```python
from build123d import *

# Parameters (mm, degrees)
MASS_DEPTH         = 6.35
SKETCH4_R          = 3.175
CUT_EXTRUDE1_DEPTH = 73.574972012
SKETCH3_W          = 12.7
SKETCH3_H          = 12.7
CUT_EXTRUDE2_DEPTH = 73.574972012
LPATTERN1_COUNT    = 3
LPATTERN1_PITCH    = 25.4


with BuildPart() as part:
    # Sketch1 → Mass (new body)
    with BuildSketch(Plane.XY):
        with BuildLine():
            Line((-44.45, -23.8125), (44.45, -23.8125))
            Line((44.45, -23.8125), (44.45, 23.8125))
            Line((44.45, 23.8125), (-44.45, 23.8125))
            ThreePointArc((-44.45, 23.8125), (-68.2625, 0), (-44.45, -23.8125))
        make_face()
    extrude(amount=MASS_DEPTH)

    # Sketch4 → Cut-Extrude1 (cut, through all)
    with BuildSketch(Plane(origin=(0, 0, 0), x_dir=(-1, 0, 0), z_dir=(0, 0, -1))):
        with Locations((44.45, 0)):
            Circle(SKETCH4_R)
    extrude(amount=-CUT_EXTRUDE1_DEPTH, mode=Mode.SUBTRACT)

    # Sketch3 → Cut-Extrude2 (cut, through all)
    with BuildSketch(Plane(origin=(0, 0, 0), x_dir=(-1, 0, 0), z_dir=(0, 0, -1))):
        with Locations((-25.4, 23.8125)):
            Rectangle(SKETCH3_W, SKETCH3_H)
        with Locations((-25.4, -23.8125)):
            Rectangle(SKETCH3_W, SKETCH3_H)
    cut_extrude2 = extrude(amount=-CUT_EXTRUDE2_DEPTH, mode=Mode.SUBTRACT)

    # LPattern1: Cut-Extrude2 ×3
    with Locations(*[(-i * LPATTERN1_PITCH, 0, 0) for i in range(1, LPATTERN1_COUNT)]):
        add(cut_extrude2, mode=Mode.SUBTRACT)


solid = part.part
```
Check sheet for the modelled part. Datum: model origin and axes. Units: mm. A direction names the side the tool comes from. Round coordinates to 2 decimals unless told otherwise and drop trailing zeros. Loops run counter-clockwise (first coordinate to the right, second up) from the corner with the lowest first, then second, coordinate; pieces in that order, holes last. Notation, with made-up numbers: (84, 82) - (118, 82) arc R15 ccw to (118, 107) - close; hole circle Ø8 at (12.5, -5.5). An arc over 180 degrees is marked (long way). Answer as a JSON object with one key per item and string values. Group by question number.
Q1. Set-up check for faces 1 (the face through (-38, 23.812, 3)), 2 (the face through (0, 17.462, 3)), 3 (the face through (6.35, -21, 3)): record each of +Z, -Z, +X, -X, +Y, -Y from which the full face is reachable in a straight line by a thin tool's end or side.
Q2. Sectioned sample at C-C, the plane x = -43. Enter the section's corners in (y, z), plus the area to 3 significant figures.
Q3. Scan lines: line 1 along Y through (x, z) = (-44.45, 3.75) (1 decimal); line 2 along X through (y, z) = (-21.5, 2.5); line 3 along Y through (x, z) = (23, 2). Record each from-to range of solid material in increasing order. Write a range as [from, to].
Q4. Gauge pin test, flat ends, axial feed: P1, Ø3, axis at x = 24.5, z = 4.5, coming from the +Y side; P2, Ø1.9, axis at y = -21, z = 4, coming from the -X side; P3, Ø3, axis at y = -22, z = 4, coming from the -X side. Record the tip position at first contact, or that the pin passes through.
Q5. Sectioned sample at D-D, the plane y = -18.5. Enter the section's corners in (x, z).
Q6. Mould release check, pull along X, two halves, no side actions. Record for faces 4 (the face through (-13, 0, 0)), 5 (the face through (-19.05, 21, 3)), 6 (the face through (-68.257, 0.524, 3.131)), 7 (the face through (-19.05, -21, 3)): released by +X, released by -X, zero draft, split by the parting line, or undercut.
Solution:
{
 "1": {"face 1": "+Z, -Z, +X, -X, +Y", "face 2": "+Z, -Z, +Y", "face 3": "+Z, -Z, -Y"},
 "2": {"outline": "(-23.81, 0) - (-2.82, 0) - (-2.82, 6.35) - (-23.81, 6.35) - close; (2.82, 0) - (23.81, 0) - (23.81, 6.35) - (2.82, 6.35) - close", "area": "267 mm²"},
 "3": {"line 1": "y = [-23.8, -3.2], [3.2, 23.8]", "line 2": "x = [-54.69, -31.75], [-19.05, -6.35], [6.35, 19.05], [31.75, 44.45]", "line 3": "y = [-17.46, 17.46]"},
 "4": {"P1": "stops at y = 17.46", "P2": "stops at x = -57.3", "P3": "stops at x = -56.57"},
 "5": {"outline": "(-59.44, 0) - (-31.75, 0) - (-31.75, 6.35) - (-59.44, 6.35) - close; (-19.05, 0) - (-6.35, 0) - (-6.35, 6.35) - (-19.05, 6.35) - close; (6.35, 0) - (19.05, 0) - (19.05, 6.35) - (6.35, 6.35) - close; (31.75, 0) - (44.45, 0) - (44.45, 6.35) - (31.75, 6.35) - close"},
 "6": {"face 4": "zero draft", "face 5": "undercut", "face 6": "released by -X", "face 7": "undercut"}
}
